from build123d import *

# Parameters (mm, degrees)
SKETCH_1_R          = 6.1
SKETCH_1_R_2        = 5.1
EXTRUDE_1_DEPTH     = 11
SKETCH_2_R          = 17.5
SKETCH_2_R_2        = 5.1
EXTRUDE_2_DEPTH     = 5
SKETCH_4_OUTSIDE_W  = 47.754
SKETCH_4_OUTSIDE_H  = 47.754
SKETCH_4_OUTSIDE_R  = 16.5
CUT_EXTRUDE_1_DEPTH = 33.457664734


with BuildPart() as part:
    # 스케치1 → 보스-돌출1 (new body)
    with BuildSketch(Plane.XY):
        Circle(SKETCH_1_R)
        Circle(SKETCH_1_R_2, mode=Mode.SUBTRACT)
    extrude(amount=EXTRUDE_1_DEPTH)

    # 스케치2 → 보스-돌출2 (add)
    with BuildSketch(Plane.XY.offset(11)):
        Circle(SKETCH_2_R)
        Circle(SKETCH_2_R_2, mode=Mode.SUBTRACT)
    extrude_2 = extrude(amount=EXTRUDE_2_DEPTH)

    # 대칭 복사1: 보스-돌출2 across plane
    add(extrude_2.mirror(Plane.XY.offset(5.5)))

    # 스케치3 → 컷-회전1 (revolve, cut)
    with BuildSketch(Plane(origin=(0, 0, 0), x_dir=(1, 0, 0), z_dir=(0, 1, 0))):
        Polygon((-17.5, 5), (-6.1, 0), (-17.5, 0), align=None)
        Polygon((-17.5, -11), (-17.5, -16), (-6.1, -11), align=None)
    revolve(axis=Axis((0, 0, -9.433987915), (0, 0, 1)), mode=Mode.SUBTRACT)

    # 스케치4 outside → 컷-돌출1 (cut, through all)
    with BuildSketch(Plane.XY.offset(16)):
        Rectangle(SKETCH_4_OUTSIDE_W, SKETCH_4_OUTSIDE_H)
        Circle(SKETCH_4_OUTSIDE_R, mode=Mode.SUBTRACT)
    extrude(amount=-CUT_EXTRUDE_1_DEPTH, mode=Mode.SUBTRACT)


solid = part.part
Geometry: final body of the model. Coordinates: model frame, mm. A direction names the side the tool comes from. Give positions to 0.01 mm unless a question says otherwise; leave off trailing zeros. Write each loop counter-clockwise with the first axis right and the second up, starting at its lowest first coordinate (ties: lowest second). Pieces come first, ordered by that corner, then holes.
(1) Mould query, pull axis Z, two halves, no side actions, for faces 3 (the conical face through (-3.05, 5.86, 11.22)), 4 (the cylindrical face through (-3.577, -16.108, 15.784)), 5 (the flat face through (-4, 4, -5)). Classes: released by +Z, released by -Z, zero draft, split by the parting line, or undercut.
(2) Cut plane C-C, the plane z = 4. Return loops of the section in (x, y).
(3) Cut plane A-A, the plane y = 0. Return loops of the section in (x, z).
(4) Cut plane D-D, the plane z = 14.5. Return loops of the section in (x, y).
(5) Ray query, line 1 (Y direction, x = 0, z = 5.25); line 2 (Z direction, x = -14.5, y = 4.5); line 3 (Z direction, x = 5, y = -11.5). Return the intervals inside material, ascending.
(6) First-contact query: P1, Ø1, axis at y = -4.5, z = 10, coming from the -X side; P2, Ø1, axis at y = -2, z = 11.5, coming from the -X side. Flat tips, straight axial feed; report the tip coordinate or a pass-through.
(7) Access query for faces 1 (the flat face through (-4, 4, 16)), 2 (the conical face through (-3.05, 5.86, -0.22)). Directions: +Z, -Z, +X, -X, +Y, -Y. A direction counts if a zero-diameter tool reaches every point of the face in a straight line with its end or side. Return the directions, or none.
Values follow:
1. face 3: undercut
1. face 4: zero draft
1. face 5: released by -Z
2. outline: circle Ø12.2 at (0, 0); hole circle Ø10.2 at (0, 0)
3. outline: (-16.5, -5) - (-5.1, -5) - (-5.1, 16) - (-16.5, 16) - (-16.5, 15.56) - (-6.1, 11) - (-6.1, 0) - (-16.5, -4.56) - close; (5.1, -5) - (16.5, -5) - (16.5, -4.56) - (6.1, 0) - (6.1, 11) - (16.5, 15.56) - (16.5, 16) - (5.1, 16) - close
4. outline: circle Ø28.16 at (0, 0); hole circle Ø10.2 at (0, 0)
5. line 1: y = -6.1 to -5.1, 5.1 to 6.1
5. line 2: z = -5 to -3.98, 14.98 to 16
5. line 3: z = -5 to -2.82, 13.82 to 16
6. P1: stops at x = -4.61
6. P2: stops at x = -8.14
7. face 1: +Z, +X, -X, +Y, -Y
7. face 2: none
